```python
from build123d import *

# Parameters (mm, degrees)
F0_W     = 1220
F0_H     = 515
F1_DEPTH = 20
F2_W     = 1200
F2_H     = 8
F3_DEPTH = 30
F4_W     = 8
F4_H     = 492
F5_DEPTH = 30
F6_W     = 8
F6_H     = 492
F7_DEPTH = 30
F8_ANGLE = 180


with BuildPart() as f1:
    # F0 (on Top) → F1 (new body, symmetric)
    with BuildSketch(Plane.XY):
        Rectangle(F0_W, F0_H)
    extrude(amount=F1_DEPTH, both=True)

    # F2 (on face) → F3 (cut)
    with BuildSketch(Plane.XY.offset(20)):
        with Locations((0, 243.5)):
            Rectangle(F2_W, F2_H)
    extrude(amount=-F3_DEPTH, mode=Mode.SUBTRACT)

    # F4 (on face) → F5 (cut)
    with BuildSketch(Plane.XY.offset(20)):
        with Locations((-596, 1.5)):
            Rectangle(F4_W, F4_H)
    extrude(amount=-F5_DEPTH, mode=Mode.SUBTRACT)

    # F6 (on face) → F7 (cut)
    with BuildSketch(Plane.XY.offset(20)):
        with Locations((596, -6.5)):
            Rectangle(F6_W, F6_H)
    extrude(amount=-F7_DEPTH, mode=Mode.SUBTRACT)


with BuildPart() as f1_1:
    # F8: moved
    add(f1.part.rotate(Axis((-610, 0, 20), (0, 1, 0)), F8_ANGLE))


solid = f1_1.part
```
CAD build for the part. Positions are in the model's coordinates, mm. A direction names the side the tool comes from. Round coordinates to 2 decimals unless told otherwise and drop trailing zeros. Write each loop counter-clockwise with the first axis right and the second up, starting at its lowest first coordinate (ties: lowest second). Pieces come first, ordered by that corner, then holes. Notation, with made-up numbers: (86, -5) - (95, -5) arc R32 cw to (95, 31) - close; hole circle Ø11 at (-17.5, 88.25). An arc over 180 degrees is marked (long way). Return JSON: item names as keys, results as strings. Group by question number.
Item 1: Band-saw the part on A-A on z = 35. List the corners of the cut face in (x, y), plus the area to 3 significant figures.
Item 2: Mould opens along Y. For faces 3 (the face through (-620, -2, 35)), 4 (the face through (-1211, -257.5, 40)), 5 (the face through (-628, -6, 35)), 6 (the face through (-1211, 4, 20)) say: +Y half, -Y half, draft (parallel to the pull), parting line (faces both ways), or undercut.
Item 3: 3-axis set-ups, long thin cutter, end or side, ignore diameter. For faces 1 (the face through (-1211, 4, 60)), 2 (the face through (-1820, -6, 35)): which of +Z, -Z, +X, -X, +Y, -Y reach the whole face in a straight line?
Item 4: Probe probe 1 along X at (y, z) = (-128, 23.5); probe 2 along Y at (x, z) = (-1594.5, 35). List the from-to ranges inside material, lowest first.
Resolved:
{
 "1": {"outline": "(-1830, -257.5) - (-610, -257.5) - (-610, 257.5) - (-1830, 257.5) - close; hole (-1820, -252.5) - (-1812, -252.5) - (-1812, 239.5) - (-628, 239.5) - (-628, -244.5) - (-620, -244.5) - (-620, 247.5) - (-1820, 247.5) - close", "area": "611,000 mm²"},
 "2": {"face 3": "undercut", "face 4": "-Y half", "face 5": "undercut", "face 6": "draft"},
 "3": {"face 1": "+Z, +X, -X, +Y, -Y", "face 2": "-Z"},
 "4": {"probe 1": "x = -1830 to -1820, -1812 to -628, -620 to -610", "probe 2": "y = -257.5 to 239.5, 247.5 to 257.5"}
}
